Model file for the job. Use its own axes, mm. Give positions to 0.01 mm unless a question says otherwise; leave off trailing zeros. Write each loop counter-clockwise with the first axis right and the second up, starting at its lowest first coordinate (ties: lowest second). Pieces come first, ordered by that corner, then holes. Notation, with made-up numbers: M 56,62.5 L 83,62.5 A15 cw 83,79.5 Z; hole C 9,85.25 d6. An arc over 180 degrees is marked long. Answer as a JSON object with one key per item and string values. Group by question number.
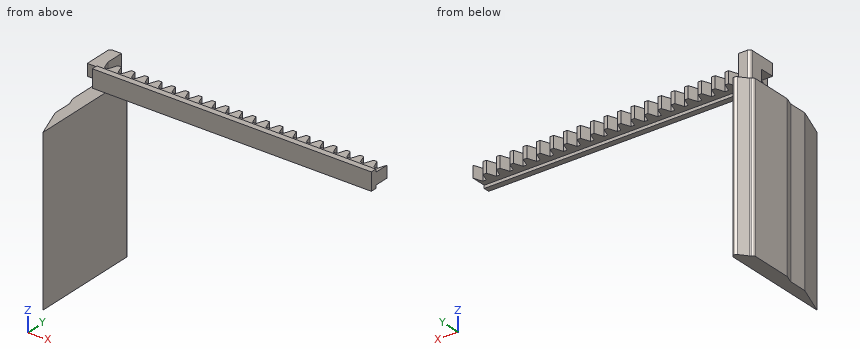
```python
from build123d import *

# Parameters (mm, degrees)
BOSS_EXTRU_2_DEPTH      = 4
ESQUISSE5_W             = 1
ESQUISSE5_H             = 2
BOSS_EXTRU_3_DEPTH      = 95
ESQUISSE6_W             = 4
ESQUISSE6_H             = 10
BOSS_EXTRU_4_DEPTH      = 4
ESQUISSE7_W             = 10
ESQUISSE7_H             = 5
BOSS_EXTRU_5_DEPTH      = 4
BOSS_EXTRU_6_DEPTH      = 50
BOSS_EXTRU_6_DEPTH_BACK = 5
CONG_1_R                = 1
CONG_2_R                = 1


with BuildPart() as part:
    # Esquisse2 → Boss.-Extru.2 (new body)
    with BuildSketch(Plane.XY):
        Polygon((-0.6, 0), (0.6, 0), (1.691910703, 3), (2.891910703, 3), (3.983821406, 0), (5.183821406, 0), (6.275732108, 3), (7.475732108, 3), (8.567642811, 0), (9.767642811, 0), (10.859553514, 3), (12.059553514, 3), (13.151464217, 0), (14.351464217, 0), (15.44337492, 3), (16.64337492, 3), (17.735285622, 0), (18.935285622, 0), (20.027196325, 3), (21.227196325, 3), (22.319107028, 0), (23.519107028, 0), (24.611017731, 3), (25.811017731, 3), (26.902928434, 0), (28.102928434, 0), (29.194839136, 3), (30.394839136, 3), (31.486749839, 0), (32.686749839, 0), (33.778660542, 3), (34.978660542, 3), (36.070571245, 0), (37.270571245, 0), (38.362481948, 3), (39.562481948, 3), (40.65439265, 0), (41.85439265, 0), (42.946303353, 3), (44.146303353, 3), (45.238214056, 0), (46.438214056, 0), (47.5, 3.000064821), (47.5, -4), (-47.5, -4), (-47.5, 3), (-46.4210099, -0.004671254), (-45.221021012, -0.009835451), (-44.116209929, 2.985437734), (-42.916209929, 2.985437734), (-41.824299226, -0.014562266), (-40.624299226, -0.014562266), (-39.532388523, 2.985437734), (-38.332388523, 2.985437734), (-37.24047782, -0.014562266), (-36.04047782, -0.014562266), (-34.948567118, 2.985437734), (-33.748567118, 2.985437734), (-32.656656415, -0.014562266), (-31.456656415, -0.014562266), (-30.364745712, 2.985437734), (-29.164745712, 2.985437734), (-28.072835009, -0.014562266), (-26.872835009, -0.014562266), (-25.780924306, 2.985437734), (-24.580924306, 2.985437734), (-23.489013604, -0.014562266), (-22.289013604, -0.014562266), (-21.197102901, 2.985437734), (-19.997102901, 2.985437734), (-18.905192198, -0.014562266), (-17.705192198, -0.014562266), (-16.613281495, 2.985437734), (-15.413281495, 2.985437734), (-14.321370793, -0.014562266), (-13.121370793, -0.014562266), (-12.02946009, 2.985437734), (-10.82946009, 2.985437734), (-9.737549387, -0.014562266), (-8.537549387, -0.014562266), (-7.445638684, 2.985437734), (-6.245638684, 2.985437734), (-5.153727981, -0.014562266), (-3.953727981, -0.014562266), (-2.891910703, 3), (-1.691910703, 3), align=None)
    extrude(amount=-BOSS_EXTRU_2_DEPTH)

    # Esquisse5 → Boss.-Extru.3 (add)
    with BuildSketch(Plane.ZY.offset(47.5)):
        with Locations((0.5, -3)):
            Rectangle(ESQUISSE5_W, ESQUISSE5_H)
        with Locations((-4.5, -3)):
            Rectangle(ESQUISSE5_W, ESQUISSE5_H)
    extrude(amount=-BOSS_EXTRU_3_DEPTH)

    # Esquisse6 → Boss.-Extru.4 (add)
    with BuildSketch(Plane(origin=(0, 0, -4), x_dir=(-1, 0, 0), z_dir=(0, 0, -1))):
        with Locations((49.5, 4.006649999)):
            Rectangle(ESQUISSE6_W, ESQUISSE6_H)
    extrude(amount=-BOSS_EXTRU_4_DEPTH)

    # Esquisse7 → Boss.-Extru.5 (add)
    with BuildSketch(Plane.ZY.offset(51.5)):
        with Locations((-9, 6.506649999)):
            Rectangle(ESQUISSE7_W, ESQUISSE7_H)
    extrude(amount=-BOSS_EXTRU_5_DEPTH)

    # Esquisse8 → Boss.-Extru.6 (add, two sides: drawn at the far end of the back side and taken through both)
    with BuildSketch(Plane(origin=(0, 0, -14), x_dir=(-1, 0, 0), z_dir=(0, 0, -1)).offset(-BOSS_EXTRU_6_DEPTH_BACK)):
        Polygon((47.5, 14.006649999), (47.5, -25.993350001), (51.5, -15.317080155), (51.5, -8.917080155), (52.5, -6.248012693), (52.5, 8.631987307), (51.5, 9.006649999), align=None)
    extrude(amount=BOSS_EXTRU_6_DEPTH + BOSS_EXTRU_6_DEPTH_BACK)

    # Congé1
    # the kernel refuses this fillet: 1 mm, written as the material it adds along each edge
    with BuildSketch(Plane(origin=(-51.5, 9.006649999, -9), x_dir=(0.6246950475544211, 0.7808688094430328, 0), z_dir=(0, 0, -1))) as cong_1_piece_1:
        with BuildLine():
            CenterArc((CONG_1_R * 0.275456143741, -CONG_1_R), CONG_1_R, 90, 30.801092038)
            Line((-CONG_1_R * 0.236603092518, -CONG_1_R * 0.141049862587), (0, 0))
            Line((0, 0), (CONG_1_R * 0.275456143741, 0))
        make_face()
    extrude(amount=55)
    with BuildSketch(Plane(origin=(-51.5, -8.917080155, -9), x_dir=(-0.35084650222761954, 0.9364329831197985, 0), z_dir=(0, 0, -1))) as cong_1_piece_2:
        with BuildLine():
            CenterArc((CONG_1_R * 0.18118184584, -CONG_1_R), CONG_1_R, 90, 20.539099708)
            Line((-CONG_1_R * 0.169664656387, -CONG_1_R * 0.0635670168802), (0, 0))
            Line((0, 0), (CONG_1_R * 0.18118184584, 0))
        make_face()
    extrude(amount=55)
    # the kernel refuses this fillet: 1 mm, written as the material it takes off along each edge
    with BuildSketch(Plane(origin=(-47.5, 14.006649999, -71.126952648), x_dir=(0, -1, 0), z_dir=(0, 0, 1))) as cong_1_2_piece_1:
        with BuildLine():
            CenterArc((CONG_1_R * 2.85078105936, -CONG_1_R), CONG_1_R, 90, 141.340191746)
            Line((CONG_1_R * 2.2260860118, -CONG_1_R * 1.78086880944), (0, 0))
            Line((0, 0), (CONG_1_R * 2.85078105936, 0))
        make_face()
    extrude(amount=69.253905297, mode=Mode.SUBTRACT)
    with BuildSketch(Plane(origin=(-52.5, 8.631987307, -65.733048465), x_dir=(0.9364329831198017, 0.35084650222761105, 0), z_dir=(0, 0, 1))) as cong_1_2_piece_2:
        with BuildLine():
            CenterArc((CONG_1_R * 0.693219386196, -CONG_1_R), CONG_1_R, 90, 69.460900292)
            Line((-CONG_1_R * 0.243213596923, -CONG_1_R * 0.649153497772), (0, 0))
            Line((0, 0), (CONG_1_R * 0.693219386196, 0))
        make_face()
    extrude(amount=58.466096931, mode=Mode.SUBTRACT)
    with BuildSketch(Plane(origin=(-52.5, -6.248012693, -8.547045385), x_dir=(0, 1, 0), z_dir=(0, 0, -1))) as cong_1_2_piece_3:
        with BuildLine():
            CenterArc((CONG_1_R * 0.18118184584, CONG_1_R), CONG_1_R, 249.460900292, 20.539099708)
            Line((-CONG_1_R * 0.169664656387, CONG_1_R * 0.0635670168802), (0, 0))
            Line((0, 0), (CONG_1_R * 0.18118184584, 0))
        make_face()
    extrude(amount=55.905909229, mode=Mode.SUBTRACT)
    with BuildSketch(Plane(origin=(-51.5, -15.317080155, -8.547045385), x_dir=(0.35084650222762276, -0.9364329831197973, 0), z_dir=(0, 0, -1))) as cong_1_2_piece_4:
        with BuildLine():
            CenterArc((CONG_1_R * 0.18118184584, -CONG_1_R), CONG_1_R, 90, 20.539099708)
            Line((-CONG_1_R * 0.169664656387, -CONG_1_R * 0.0635670168802), (0, 0))
            Line((0, 0), (CONG_1_R * 0.18118184584, 0))
        make_face()
    extrude(amount=55.905909229, mode=Mode.SUBTRACT)

    # Congé2
    cong_2_edges = [part.edges().sort_by_distance(p)[0] for p in [
        (-51.5, 9.006649999, -4.5),
    ]]
    fillet(cong_2_edges, radius=CONG_2_R)


solid = part.part
```
Q1. Drop flat-ended pins along their axis: P1, Ø2.5, axis at x = -50, y = -15, coming from the +Z side; P2, Ø3, axis at x = -3, y = 1.5, coming from the -Z side; P3, Ø3, axis at x = -26, y = 0, coming from the +Z side. Give the stop position or say it passes through.
Q2. Slice it at B-B, the plane y = 6. Write the cut outline in (x, z), then the cut area to 3 significant figures.
Q3. Slice it at A-A, the plane z = -25. Write the cut outline in (x, y), then the cut area to 3 significant figures.
Q4. Wall check: L1, parallel to Z at x = 30, y = 2; L2, parallel to X at y = 5, z = -37; L3, parallel to X at y = -11, z = -59.5. Give the ranges that are in metal, low to high.
Q5. Slice it at C-C, the plane y = -17.5. Write the cut outline in (x, z).
Solved:
{
 "1": {"P1": "stops at z = -9", "P2": "stops at z = -4", "P3": "stops at z = 0"},
 "2": {"outline": "M -52.5,-64 L -47.5,-64 L -47.5,0 L -51.5,0 L -51.5,-9 L -52.5,-9 Z", "area": "311 mm²"},
 "3": {"outline": "M -52.5,-6.07 A1 ccw -52.44,-6.42 L -51.56,-8.75 A1 cw -51.5,-9.1 L -51.5,-15.14 A1 ccw -51.44,-15.49 L -47.5,-25.99 L -47.5,11.16 A1 ccw -49.28,11.78 L -51.33,9.22 A1 cw -51.76,8.91 L -51.85,8.88 A1 ccw -52.5,7.94 Z", "area": "143 mm²"},
 "4": {"L1": "z = -4 to 0", "L2": "x = -52.5 to -47.5", "L3": "x = -51.5 to -47.5"},
 "5": {"outline": "M -50.68,-64 L -47.5,-64 L -47.5,-9 L -50.68,-9 Z"}
}
